The drawing under review shows one solid part. Ordinate dimensions are in mm from its lowest x, y, z. A direction names the side the tool comes from. Give positions to 0.01 mm unless a question says otherwise; leave off trailing zeros. Order: outer loops, then holes, each group sorted by start corner. A loop starts at its lowest first (then second) coordinate and runs counter-clockwise, first axis right, second up. Notation, with made-up numbers: (11, 42) -> (31, 42) arc R27 cw to (31, 79) -> close; hole circle Ø9 at (4.5, 76). An arc over 180 degrees is marked (long way). Return JSON: item names as keys, results as strings. Group by question number.
1) To check wall thickness, follow line 1 along Y through (x, z) = (40, 5); line 2 along X through (y, z) = (26.5, 49.5). State the ranges of each line that lie inside material, in increasing order.
2) Insertion check: P1, Ø3, axis at y = 15, z = 67.5, coming from the +X side; P2, Ø8, axis at x = 40, y = 45, coming from the +Z side; P3, Ø17.5, axis at x = 30, y = 21, coming from the +Z side. Each pin has a flat end and moves straight along its axis. Give the tip position at first contact, or say it passes through.
3) Add section B-B (x = 40). Give the boundary of the cut face in (y, z), then the cut area to 3 significant figures.
4) For the marked faces 1 and 2, list the 3-axis set-ups (+Z, -Z, +X, -X, +Y, -Y) from which the entire face can be reached by the end or side of a thin tool; tool diameter is ignored.
5) Add section C-C (y = 15). Give the boundary of the cut face in (x, z), then the cut area to 3 significant figures.
6) Add section A-A (z = 73). Give the boundary of the cut face in (x, y), then the cut area to 3 significant figures.
7) Add section D-D (y = 30). Give the boundary of the cut face in (x, z), then the cut area to 3 significant figures.
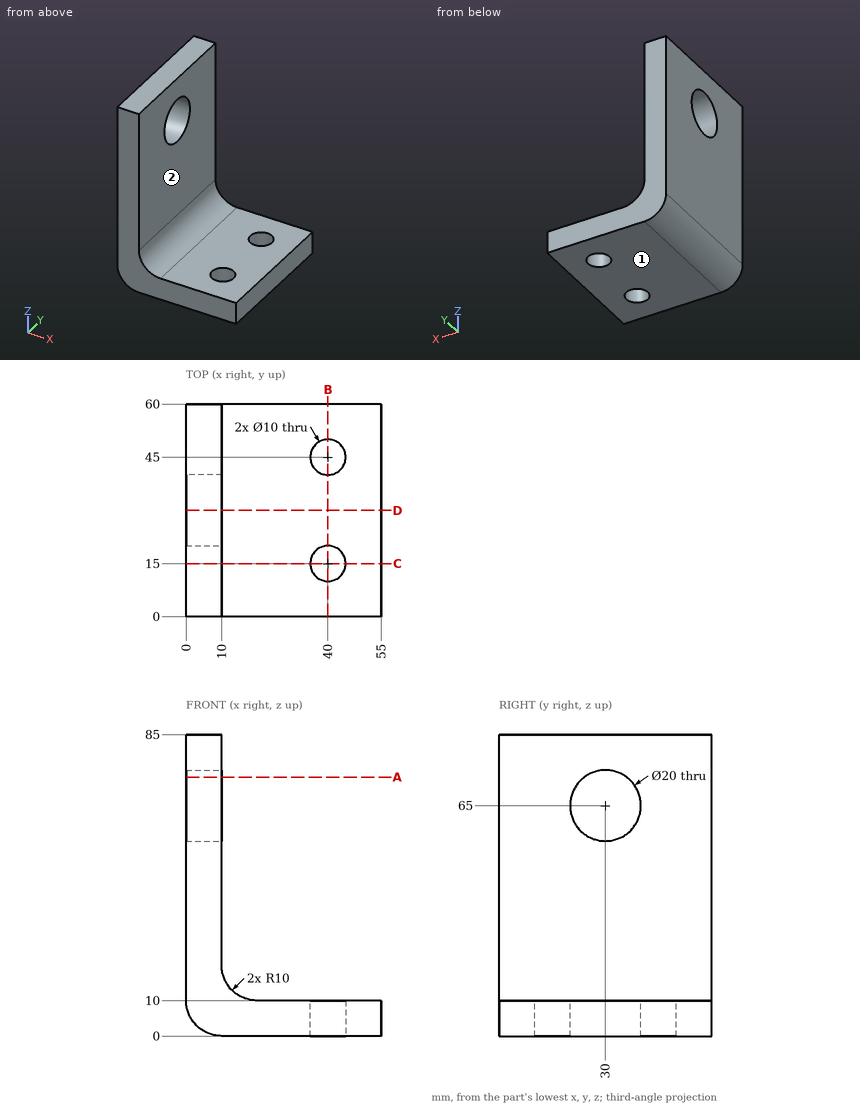
Evaluation:
{
 "1": {"line 1": "0 to 10, 20 to 40, 50 to 60", "line 2": "0 to 10"},
 "2": {"P1": "x = 10", "P2": "through", "P3": "z = 10"},
 "3": {"outline": "(0, 0) -> (10, 0) -> (10, 10) -> (0, 10) -> close; (20, 0) -> (40, 0) -> (40, 10) -> (20, 10) -> close; (50, 0) -> (60, 0) -> (60, 10) -> (50, 10) -> close", "area": "400 mm^2"},
 "4": {"face 1": "-Z, +X, -X, +Y, -Y", "face 2": "+Z, +X, +Y, -Y"},
 "5": {"outline": "(0, 10) arc R10 ccw to (10, 0) -> (35, 0) -> (35, 10) -> (20, 10) arc R10 cw to (10, 20) -> (10, 85) -> (0, 85) -> close; (45, 0) -> (55, 0) -> (55, 10) -> (45, 10) -> close", "area": "1,200 mm^2"},
 "6": {"outline": "(0, 0) -> (10, 0) -> (10, 24) -> (0, 24) -> close; (0, 36) -> (10, 36) -> (10, 60) -> (0, 60) -> close", "area": "480 mm^2"},
 "7": {"outline": "(0, 10) arc R10 ccw to (10, 0) -> (55, 0) -> (55, 10) -> (20, 10) arc R10 cw to (10, 20) -> (10, 55) -> (0, 55) -> close; (0, 75) -> (10, 75) -> (10, 85) -> (0, 85) -> close", "area": "1,100 mm^2"}
}
